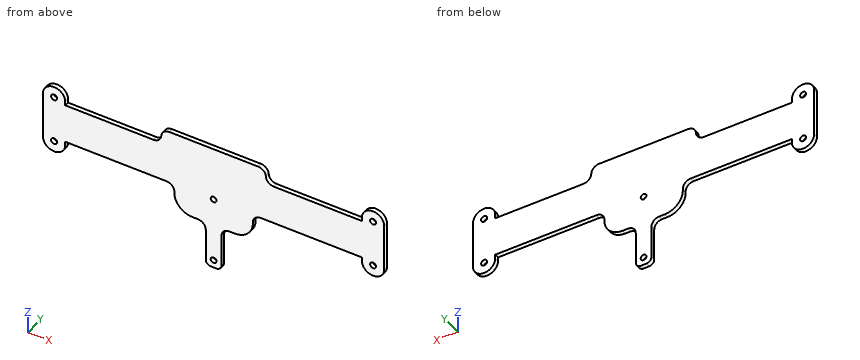
from build123d import *

# Parameters (mm, degrees)
SZKIC1_R                    = 1.15
SZKIC1_R_2                  = 1.150012437
SZKIC1_R_3                  = 1.1
DODANIE_WYCI_GNI_CIE1_DEPTH = 1.7


with BuildPart() as part:
    # Szkic1 → Dodanie-wyciągnięcie1 (new body)
    with BuildSketch(Plane.XZ.offset(-7.087491716)):
        with BuildLine():
            Line((-166.869010382, 45.27), (-166.869010382, 48.27))
            ThreePointArc((-166.869010382, 48.27), (-162.619010382, 52.52), (-158.369010382, 48.27))
            Line((-158.369010382, 48.27), (-158.369010382, 46.77))
            Line((-158.369010382, 46.77), (-124.668997945, 46.77))
            ThreePointArc((-124.668997945, 46.77), (-122.547677602, 47.648679656), (-121.668997945, 49.77))
            Line((-121.668997945, 49.77), (-121.668997945, 49.52))
            ThreePointArc((-121.668997945, 49.52), (-120.790318289, 51.641320344), (-118.668997945, 52.52))
            Line((-118.668997945, 52.52), (-84.668997945, 52.52))
            ThreePointArc((-84.668997945, 52.52), (-82.547677602, 51.641320344), (-81.668997945, 49.52))
            Line((-81.668997945, 49.52), (-81.668997945, 49.77))
            ThreePointArc((-81.668997945, 49.77), (-80.790318289, 47.648679656), (-78.668997945, 46.77))
            Line((-78.668997945, 46.77), (-44.968985509, 46.77))
            Line((-44.968985509, 46.77), (-44.968985509, 48.27))
            ThreePointArc((-44.968985509, 48.27), (-40.718985509, 52.52), (-36.468985509, 48.27))
            Line((-36.468985509, 48.27), (-36.468985509, 45.27))
            Line((-36.468985509, 45.27), (-36.468985509, 33.27))
            Line((-36.468985509, 33.27), (-36.468985509, 30.27))
            ThreePointArc((-36.468985509, 30.27), (-40.718985509, 26.02), (-44.968985509, 30.27))
            Line((-44.968985509, 30.27), (-44.968985509, 31.77))
            Line((-44.968985509, 31.77), (-83.668997945, 31.77))
            ThreePointArc((-83.668997945, 31.77), (-85.790318289, 30.891320344), (-86.668997945, 28.77))
            Line((-86.668997945, 28.77), (-86.668997945, 28.17))
            ThreePointArc((-86.668997945, 28.17), (-88.719250477, 23.220252532), (-93.668997945, 21.17))
            Line((-93.668997945, 21.17), (-95.668997945, 21.17))
            ThreePointArc((-95.668997945, 21.17), (-97.790318289, 20.291320344), (-98.668997945, 18.17))
            Line((-98.668997945, 18.17), (-98.668997945, 5.82))
            ThreePointArc((-98.668997945, 5.82), (-99.254784383, 4.405786438), (-100.668997945, 3.82))
            Line((-100.668997945, 3.82), (-102.668997945, 3.82))
            ThreePointArc((-102.668997945, 3.82), (-104.083211508, 4.405786438), (-104.668997945, 5.82))
            Line((-104.668997945, 5.82), (-104.668997945, 18.17))
            ThreePointArc((-104.668997945, 18.17), (-105.547677602, 20.291320344), (-107.668997945, 21.17))
            Line((-107.668997945, 21.17), (-109.668997945, 21.17))
            ThreePointArc((-109.668997945, 21.17), (-114.618745414, 23.220252532), (-116.668997945, 28.17))
            Line((-116.668997945, 28.17), (-116.668997945, 28.77))
            ThreePointArc((-116.668997945, 28.77), (-117.547677602, 30.891320344), (-119.668997945, 31.77))
            Line((-119.668997945, 31.77), (-158.369010382, 31.77))
            Line((-158.369010382, 31.77), (-158.369010382, 30.27))
            ThreePointArc((-158.369010382, 30.27), (-162.619010382, 26.02), (-166.869010382, 30.27))
            Line((-166.869010382, 30.27), (-166.869010382, 33.27))
            Line((-166.869010382, 33.27), (-166.869010382, 45.27))
        make_face()
        with Locations((-162.618997945, 30.27)):
            Circle(SZKIC1_R, mode=Mode.SUBTRACT)
        with Locations((-162.618997945, 48.27)):
            Circle(SZKIC1_R, mode=Mode.SUBTRACT)
        with Locations((-40.718985509, 48.27)):
            Circle(SZKIC1_R_2, mode=Mode.SUBTRACT)
        with Locations((-40.718985509, 30.27)):
            Circle(SZKIC1_R_2, mode=Mode.SUBTRACT)
        with Locations((-101.668997945, 31.82)):
            Circle(SZKIC1_R_3, mode=Mode.SUBTRACT)
        with Locations((-101.668997945, 6.82)):
            Circle(SZKIC1_R_3, mode=Mode.SUBTRACT)
    extrude(amount=DODANIE_WYCI_GNI_CIE1_DEPTH)


solid = part.part
Model file for the job. Use its own axes, mm. Give positions to 0.01 mm unless a question says otherwise; leave off trailing zeros. Write each loop counter-clockwise with the first axis right and the second up, starting at its lowest first coordinate (ties: lowest second). Pieces come first, ordered by that corner, then holes. Notation, with made-up numbers: (-35, -8) -> (10, -8) arc R31 cw to (10, 27) -> close; hole circle Ø2 at (-30, -5). An arc over 180 degrees is marked (long way). Write item = value, one per line.
(1) Slice it at B-B, the plane z = 13. Give the cut face in (x, y).
Determined:
outline = (-104.67, 5.39) -> (-98.67, 5.39) -> (-98.67, 7.09) -> (-104.67, 7.09) -> close
(2) Slice it at A-A, the plane y = 6.7. Give the number of separate pieces and of enclosed holes in the cut face, then the cut area to 3 significant figures.
Determined:
separate_pieces = 1
enclosed_holes = 6
area = 2,730 mm2
(3) Probe line 1 along X through (y, z) = (6.05, 30); line 2 along X through (y, z) = (5.65, 8); line 3 along Z through (x, y) = (-61, 6.7). List the from-to ranges inside material, lowest first.
Determined:
line_1 = -166.86 to -163.74, -161.5 to -158.38, -116.93 to -86.41, -44.96 to -41.84, -39.6 to -36.48
line_2 = -104.67 to -98.67
line_3 = 31.77 to 46.77
(4) Flat gauge pins, fed straight in: P1, Ø1, axis at x = -135.5, y = 6.5, coming from the +Z side; P2, Ø0.5, axis at x = -129.5, y = 6.5, coming from the -Z side; P3, Ø0.5, axis at y = 6, z = 11, coming from the +X side. Where does each tip first touch, or does it go through?
Determined:
P1 = 46.77
P2 = 31.77
P3 = -98.67
(5) Slice it at C-C, the plane x = -55. Give the cut face in (y, z), then the cut area to 3 significant figures.
Determined:
outline = (5.39, 31.77) -> (7.09, 31.77) -> (7.09, 46.77) -> (5.39, 46.77) -> close
area = 25.5 mm2
